Work out the finished part from the listing and answer in its coordinate system (mm). A direction names the side the tool comes from. Round coordinates to 2 decimals unless told otherwise and drop trailing zeros. Loops run counter-clockwise (first coordinate to the right, second up) from the corner with the lowest first, then second, coordinate; pieces in that order, holes last. Notation, with made-up numbers: (45.25, 49.25) - (85.25, 49.25) arc R34 cw to (85.25, 79.25) - close; hole circle Ø3 at (10, 12.25). An arc over 180 degrees is marked (long way). Use CSV: the item, a comma, the result in double quotes. Start each with the question number.
from build123d import *

# Parameters (mm, degrees)
SKETCH1_R           = 1.0500000000000007
SKETCH1_R_2         = 1.0499999999999996
SKETCH1_R_3         = 1.049999999999999
SKETCH1_R_4         = 1.0500000000000005
BOSS_EXTRUDE2_DEPTH = 1
BOSS_EXTRUDE4_START = 3
BOSS_EXTRUDE4_DEPTH = 3
BOSS_EXTRUDE5_DEPTH = 8


with BuildPart() as part:
    # Sketch1 → Boss-Extrude2 (new body)
    with BuildSketch(Plane(origin=(0, 0, 0), x_dir=(1, 0, 0), z_dir=(0, 1, 0))):
        with BuildLine():
            ThreePointArc((-10.499999999999952, -8.649999999999997), (-11.808147545195132, -11.80814754519509), (-8.650000000000002, -10.499999999999996))
            Line((-8.65, -10.499999999999996), (13.149999999999997, -10.499999999999979))
            ThreePointArc((13.149999999999999, -10.499999999999913), (16.308147545195062, -11.808147545195157), (15.000000000000048, -8.649999999999997))
            Line((15.000000000000046, -8.649999999999997), (14.999999999999996, 13.15))
            ThreePointArc((15.000000000000046, 13.150000000000002), (16.308147545195123, 16.3081475451951), (13.149999999999999, 15.000000000000085))
            Line((13.149999999999999, 15.000000000000021), (-8.649999999999999, 15.000000000000002))
            ThreePointArc((-8.65, 15.000000000000002), (-11.808147545195128, 16.308147545195098), (-10.499999999999954, 13.150000000000002))
            Line((-10.5, 13.150000000000002), (-10.5, -8.649999999999997))
        make_face()
        with Locations(Location((-10.499999999999998, -10.499999999999998, 0), (0, 0, 270))):
            Circle(SKETCH1_R, mode=Mode.SUBTRACT)
        with Locations(Location((14.999999999999998, 15.000000000000002, 0), (0, 0, 270))):
            Circle(SKETCH1_R_2, mode=Mode.SUBTRACT)
        with Locations(Location((14.999999999999998, -10.499999999999995, 0), (0, 0, 270))):
            Circle(SKETCH1_R_3, mode=Mode.SUBTRACT)
        with Locations(Location((-10.5, 15, 0), (0, 0, 270))):
            Circle(SKETCH1_R_4, mode=Mode.SUBTRACT)
    extrude(amount=-BOSS_EXTRUDE2_DEPTH)

    # Sketch1_5 → Boss-Extrude4 (add)
    with BuildSketch(Plane(origin=(0, 0, 0), x_dir=(1, 0, 0), z_dir=(0, 1, 0)).offset(BOSS_EXTRUDE4_START)):
        with BuildLine():
            ThreePointArc((15.000000000000046, -8.649999999999997), (13.691852454804902, -9.191852454804867), (13.149999999999999, -10.499999999999996))
            Line((13.149999999999999, -10.499999999999996), (13.949999999999996, -10.499999999999996))
            ThreePointArc((13.949999999999998, -10.499999999999996), (14.257537879754121, -9.757537879754123), (14.999999999999995, -9.449999999999996))
            Line((14.999999999999998, -9.449999999999996), (14.999999999999998, -8.649999999999997))
        make_face()
        with BuildLine():
            Line((13.949999999999996, -10.499999999999996), (13.149999999999999, -10.499999999999996))
            ThreePointArc((13.149999999999999, -10.499999999999996), (14.999999999999998, -12.349999999999996), (16.849999999999998, -10.499999999999996))
            ThreePointArc((16.849999999999998, -10.499999999999996), (16.308147545195126, -9.1918524548049), (15.000000000000046, -8.649999999999997))
            Line((14.999999999999998, -8.649999999999997), (14.999999999999998, -9.449999999999996))
            ThreePointArc((14.999999999999995, -9.449999999999996), (15.742462120245872, -9.75753787975412), (16.049999999999997, -10.499999999999996))
            ThreePointArc((16.049999999999997, -10.499999999999996), (14.999999999999998, -11.549999999999997), (13.949999999999998, -10.499999999999996))
        make_face()
        with BuildLine():
            ThreePointArc((13.149999999999999, 15.000000000000002), (13.691852454804902, 13.691852454804874), (15.000000000000046, 13.150000000000002))
            Line((14.999999999999998, 13.150000000000002), (14.999999999999998, 13.95))
            ThreePointArc((14.999999999999995, 13.950000000000001), (14.257537879754121, 14.257537879754128), (13.949999999999998, 15.000000000000002))
            Line((13.949999999999996, 15.000000000000002), (13.149999999999999, 15.000000000000002))
        make_face()
        with BuildLine():
            Line((14.999999999999998, 13.95), (14.999999999999998, 13.150000000000002))
            ThreePointArc((15.000000000000046, 13.150000000000002), (16.308147545195126, 13.691852454804906), (16.849999999999998, 15.000000000000002))
            ThreePointArc((16.849999999999998, 15.000000000000002), (14.999999999999998, 16.85), (13.149999999999999, 15.000000000000002))
            Line((13.149999999999999, 15.000000000000002), (13.949999999999996, 15.000000000000002))
            ThreePointArc((13.949999999999998, 15.000000000000002), (14.999999999999998, 16.05), (16.049999999999997, 15.000000000000002))
            ThreePointArc((16.049999999999997, 15.000000000000002), (15.742462120245872, 14.257537879754125), (14.999999999999995, 13.950000000000001))
        make_face()
        with BuildLine():
            ThreePointArc((-10.500000000000004, -9.449999999999996), (-9.757537879754127, -9.75753787975412), (-9.45, -10.499999999999996))
            Line((-9.45, -10.499999999999996), (-8.65, -10.499999999999996))
            ThreePointArc((-8.65, -10.499999999999996), (-9.19185245480487, -9.1918524548049), (-10.499999999999952, -8.649999999999997))
            Line((-10.5, -8.649999999999997), (-10.5, -9.449999999999996))
        make_face()
        with BuildLine():
            Line((-8.65, -10.499999999999996), (-9.45, -10.499999999999996))
            ThreePointArc((-9.45, -10.499999999999996), (-11.242462120245873, -11.242462120245873), (-10.500000000000004, -9.449999999999996))
            Line((-10.5, -9.449999999999996), (-10.5, -8.649999999999997))
            ThreePointArc((-10.499999999999952, -8.649999999999997), (-11.80814754519513, -11.808147545195093), (-8.65, -10.499999999999996))
        make_face()
        with BuildLine():
            ThreePointArc((-8.65, 15.000000000000002), (-11.808147545195128, 16.308147545195098), (-10.499999999999954, 13.150000000000002))
            Line((-10.5, 13.150000000000002), (-10.5, 13.95))
            ThreePointArc((-10.500000000000004, 13.950000000000001), (-11.242462120245873, 15.742462120245879), (-9.45, 15.000000000000002))
            Line((-9.45, 15.000000000000002), (-8.65, 15.000000000000002))
        make_face()
        with BuildLine():
            Line((-10.5, 13.95), (-10.5, 13.150000000000002))
            ThreePointArc((-10.499999999999954, 13.150000000000002), (-9.191852454804872, 13.691852454804906), (-8.65, 15.000000000000002))
            Line((-8.65, 15.000000000000002), (-9.45, 15.000000000000002))
            ThreePointArc((-9.45, 15.000000000000002), (-9.757537879754127, 14.257537879754125), (-10.500000000000004, 13.950000000000001))
        make_face()
    extrude(amount=-BOSS_EXTRUDE4_DEPTH)

    # Sketch2 → Boss-Extrude5 (add)
    with BuildSketch(Plane(origin=(0, 0, 0), x_dir=(1, 0, 0), z_dir=(0, 1, 0))):
        Polygon((8.749999999999998, -4.249999999999995), (-4.250000000000001, -4.2499999999999964), (-4.250000000000001, 8.750000000000002), (8.749999999999998, 8.750000000000002), align=None)
        Polygon((7.949999999999997, -3.4499999999999953), (7.949999999999997, 7.950000000000004), (-3.450000000000001, 7.950000000000002), (-3.4500000000000015, -3.4499999999999966), align=None, mode=Mode.SUBTRACT)
    extrude(amount=BOSS_EXTRUDE5_DEPTH)


solid = part.part
Item 1: A cutting plane is placed at B-B (z = -6.25). Determine the outline of the cut face in (x, y), plus the area to 3 significant figures.
Item 2: Which of the six approach directions +Z, -Z, +X, -X, +Y, -Y give full straight-line access (tool end or side, diameter ignored) to faces 5 (the flat face through (2, 4, 4.25)), 6 (the flat face through (8.75, 4, -2)), 7 (the flat face through (2.4, -0.5, -15)), 8 (the cylindrical face through (16.364, 1.028, 11.75))?
Item 3: Find the intervals of material crossed by probe 1 along X at (y, z) = (0.8, -15); probe 2 along X at (y, z) = (5.25, -6); probe 3 along Z at (x, y) = (5.5, 4), in increasing order. Write a range as [from, to].
Item 4: A cutting plane is placed at A-A (y = -0.5). Determine the outline of the cut face in (x, z), plus the area to 3 significant figures.
Item 5: Each of these flat-tipped pins is pushed along its axis until it touches: pin 1 Ø3 at (x, z) = (-11, 11) entering from +Y; pin 2 Ø2 at (y, z) = (4, -7) entering from +X; pin 3 Ø3 at (y, z) = (2.5, 0.5) entering from -X; pin 4 Ø8 at (x, z) = (-1.5, -6) entering from +Y. Where does it stop, or does it pass through?
Item 6: The mould has two halves that part along Z. Classify faces 1 (the flat face through (7.95, 4, -2)), 2 (the flat face through (2.1, -0.5, 10.5)), 3 (the flat face through (-10.5, -0.5, -2.4)), 4 (the flat face through (-4.25, 4, -2)): pulls with the +Z half, pulls with the -Z half, needs draft (parallel to the pull), parting line crosses it, or undercut.
Item 7: A cutting plane is placed at C-C (x = -6.5). Determine the outline of the cut face in (y, z).
Item 8: A cutting plane is placed at D-D (z = -11.5). Determine the outline of the cut face in (x, y).
Result sheet:
1,outline,"(-10.5, -1) - (15, -1) - (15, 0) - (8.75, 0) - (8.75, 8) - (7.95, 8) - (7.95, 0) - (-3.45, 0) - (-3.45, 8) - (-4.25, 8) - (-4.25, 0) - (-10.5, 0) - close"
1,area,"38.3 mm^2"
2,face 5,"+Z, +X, -X, +Y"
2,face 6,"+Z, -Z, +X, +Y"
2,face 7,"-Z, +Y, -Y"
2,face 8,"+Y"
3,probe 1,"[-12.35, -11.55], [-9.45, -8.65], [13.15, 13.95], [16.05, 16.85]"
3,probe 2,"[-4.25, -3.45], [7.95, 8.75]"
3,probe 3,"[-8.75, -7.95], [3.45, 4.25]"
4,outline,"(-10.5, -13.15) arc R1.85 ccw (long way) to (-8.65, -15) - (13.15, -15) arc R1.85 ccw (long way) to (15, -13.15) - (15, 8.65) arc R1.85 ccw (long way) to (13.15, 10.5) - (-8.65, 10.5) arc R1.85 ccw (long way) to (-10.5, 8.65) - close; hole circle Ø2.1 at (-10.5, -15); hole circle Ø2.1 at (-10.5, 10.5); hole circle Ø2.1 at (15, -15); hole circle Ø2.1 at (15, 10.5)"
4,area,"669 mm^2"
5,pin 1,"y = 3"
5,pin 2,"x = 8.75"
5,pin 3,"x = -4.25"
5,pin 4,"y = 8"
6,face 1,"undercut"
6,face 2,"pulls with the +Z half"
6,face 3,"undercut"
6,face 4,"needs draft"
7,outline,"(-1, -15) - (0, -15) - (0, 10.5) - (-1, 10.5) - close"
8,outline,"(-10.5, -1) - (15, -1) - (15, 0) - (-10.5, 0) - close"
